```python
from build123d import *

# Parameters (mm, degrees)
BOSS_EXTRU_1_DEPTH                                 = 5
ESQUISSE7_W                                        = 36
ESQUISSE7_H                                        = 2
BOSS_EXTRU_2_DEPTH                                 = 35
BOSS_EXTRU_4_DEPTH                                 = 4
ESQUISSE1_3_R                                      = 6.5
ENL_V_MAT_EXTRU_2_DEPTH                            = 63.737548565
CHAMBRAGE_POUR_VIS_T_TE_HEXAGONALE_M41_D           = 4.5
CHAMBRAGE_POUR_VIS_T_TE_HEXAGONALE_M41_DEPTH       = 4
CHAMBRAGE_POUR_VIS_T_TE_HEXAGONALE_M41_CBORE_D     = 10.59
CHAMBRAGE_POUR_VIS_T_TE_HEXAGONALE_M41_CBORE_DEPTH = 3
CHAMBRAGE_POUR_VIS_T_TE_HEXAGONALE_M41_TIP         = 1.351936393
CONG_1_R                                           = 5
CONG_2_R                                           = 7


with BuildPart() as part:
    # Esquisse1 → Boss.-Extru.1 (new body)
    with BuildSketch(Plane(origin=(0, 0, 0), x_dir=(1, 0, 0), z_dir=(0, 1, 0))):
        with BuildLine():
            Line((20, 20), (-20, 20))
            Line((-20, 20), (-20, -3.067363788))
            ThreePointArc((-20, -3.067363788), (-23.03, -8), (-20, -12.932636212))
            Line((-20, -12.932636212), (-20, -20))
            Line((-20, -20), (20, -20))
            Line((20, -20), (20, -12.932636212))
            ThreePointArc((20, -12.932636212), (23.03, -8), (20, -3.067363788))
            Line((20, -3.067363788), (20, 20))
        make_face()
        with BuildLine():
            ThreePointArc((-16.580993336, -9.888233765), (-17.5, -10.1), (-18.419006664, -9.888233765))
            ThreePointArc((-18.419006664, -9.888233765), (-18.799038106, -8.75), (-19.594761741, -7.851766235))
            ThreePointArc((-19.594761741, -7.851766235), (-19.318653348, -6.95), (-18.675755077, -6.26))
            ThreePointArc((-18.675755077, -6.26), (-17.5, -6.5), (-16.324244923, -6.26))
            ThreePointArc((-16.324244923, -6.26), (-15.681346652, -6.95), (-15.405238259, -7.851766235))
            ThreePointArc((-15.405238259, -7.851766235), (-16.200961894, -8.75), (-16.580993336, -9.888233765))
        make_face(mode=Mode.SUBTRACT)
        with BuildLine():
            Line((4.596194078, -4.596194078), (0, -9.192388155))
            Line((0, -9.192388155), (-4.596194078, -4.596194078))
            ThreePointArc((-4.596194078, -4.596194078), (0, 6.5), (4.596194078, -4.596194078))
        make_face(mode=Mode.SUBTRACT)
        with BuildLine():
            ThreePointArc((18.419006664, -9.888233765), (17.5, -10.1), (16.580993336, -9.888233765))
            ThreePointArc((16.580993336, -9.888233765), (16.200961894, -8.75), (15.405238259, -7.851766235))
            ThreePointArc((15.405238259, -7.851766235), (15.681346652, -6.95), (16.324244923, -6.26))
            ThreePointArc((16.324244923, -6.26), (17.5, -6.5), (18.675755077, -6.26))
            ThreePointArc((18.675755077, -6.26), (19.318653348, -6.95), (19.594761741, -7.851766235))
            ThreePointArc((19.594761741, -7.851766235), (18.799038106, -8.75), (18.419006664, -9.888233765))
        make_face(mode=Mode.SUBTRACT)
    extrude(amount=-BOSS_EXTRU_1_DEPTH)

    # Esquisse7 → Boss.-Extru.2 (add)
    with BuildSketch(Plane.XZ.offset(5)):
        Polygon((-20, 2.243441463), (-20, -20), (-18, -20), (-18, -18), (-18, 2.243441463), align=None)
        with Locations((0, -19)):
            Rectangle(ESQUISSE7_W, ESQUISSE7_H)
        Polygon((18, -18), (18, -20), (20, -20), (20, 2.243441463), (18, 2.243441463), align=None)
    extrude(amount=BOSS_EXTRU_2_DEPTH)

    # Esquisse9 → Boss.-Extru.4 (add)
    with BuildSketch(Plane.XZ.offset(40)):
        Polygon((-20, 2.243441463), (-20, 20), (-40, 20), (-40, -20), (-20, -20), align=None)
        Polygon((40, 20), (20, 20), (20, 2.243441463), (20, -20), (40, -20), align=None)
        Polygon((0, -18), (0, 20), (-20, 20), (-20, 2.243441463), (-18, 2.243441463), (-18, -18), align=None)
        Polygon((0, -20), (0, -18), (-18, -18), (-18, 2.243441463), (-20, 2.243441463), (-20, -20), align=None)
        Polygon((18, -18), (0, -18), (0, -20), (20, -20), (20, 2.243441463), (18, 2.243441463), align=None)
        Polygon((20, 20), (0, 20), (0, -18), (18, -18), (18, 2.243441463), (20, 2.243441463), align=None)
    extrude(amount=BOSS_EXTRU_4_DEPTH)

    # Esquisse1<3> → Enlèv. mat.-Extru.2 (cut, through all)
    with BuildSketch(Plane(origin=(0, 0, 0), x_dir=(1, 0, 0), z_dir=(0, 1, 0))):
        Circle(ESQUISSE1_3_R)
        with BuildLine():
            Line((0, -9.192388155), (4.596194078, -4.596194078))
            ThreePointArc((4.596194078, -4.596194078), (0, -6.5), (-4.596194078, -4.596194078))
            Line((-4.596194078, -4.596194078), (0, -9.192388155))
        make_face()
    extrude(amount=-ENL_V_MAT_EXTRU_2_DEPTH, mode=Mode.SUBTRACT)

    # Chambrage pour vis à tête hexagonale M41
    with Locations(Plane(origin=(0, -40, 0), x_dir=(1, 0, 0), z_dir=(0, 1, 0))):
        with Locations((-32, -12), (-32, 12), (32, 12), (32, -12)):
            CounterBoreHole(CHAMBRAGE_POUR_VIS_T_TE_HEXAGONALE_M41_D / 2, CHAMBRAGE_POUR_VIS_T_TE_HEXAGONALE_M41_CBORE_D / 2, CHAMBRAGE_POUR_VIS_T_TE_HEXAGONALE_M41_CBORE_DEPTH, depth=CHAMBRAGE_POUR_VIS_T_TE_HEXAGONALE_M41_DEPTH)
            with Locations((0, 0, -(CHAMBRAGE_POUR_VIS_T_TE_HEXAGONALE_M41_DEPTH + CHAMBRAGE_POUR_VIS_T_TE_HEXAGONALE_M41_TIP / 2))):  # 118° drill point
                Cone(0, CHAMBRAGE_POUR_VIS_T_TE_HEXAGONALE_M41_D / 2, CHAMBRAGE_POUR_VIS_T_TE_HEXAGONALE_M41_TIP, mode=Mode.SUBTRACT)

    # Congé1
    cong_1_edges = [part.edges().sort_by_distance(p)[0] for p in [
        (18, -22.5, -18),
        (-18, -22.5, -18),
    ]]
    fillet(cong_1_edges, radius=CONG_1_R)

    # Congé2
    cong_2_edges = [part.edges().sort_by_distance(p)[0] for p in [
        (-20, -20, -20),
        (20, -20, -20),
        (20, -2.5, 20),
        (-20, -2.5, 20),
    ]]
    fillet(cong_2_edges, radius=CONG_2_R)


solid = part.part
```
Work out the finished part from the listing and answer in its coordinate system (mm). A direction names the side the tool comes from. Give positions to 0.01 mm unless a question says otherwise; leave off trailing zeros. Write each loop counter-clockwise with the first axis right and the second up, starting at its lowest first coordinate (ties: lowest second). Pieces come first, ordered by that corner, then holes.
(1) Flat-ended cylindrical pins translate along their axes: pin 1 Ø8 at (x, y) = (12.5, -18.5) entering from +Z; pin 2 Ø8 at (y, z) = (-25.5, -3.5) entering from +X; pin 3 Ø4 at (x, z) = (-32, -12) entering from +Y; pin 4 Ø8 at (x, y) = (-2, -27.5) entering from +Z. Find the tip coordinate at first contact, or state that the pin passes through.
Final values:
pin 1: stops at z = -16.57
pin 2: stops at x = 20
pin 3: passes through
pin 4: stops at z = -18
(2) The part is cut by section D-D on y = -22. Write down the section's boundary in (x, z).
Final values:
outline: (-20, -13) arc R7 ccw to (-13, -20) - (13, -20) arc R7 ccw to (20, -13) - (20, 2.24) - (18, 2.24) - (18, -13) arc R5 cw to (13, -18) - (-13, -18) arc R5 cw to (-18, -13) - (-18, 2.24) - (-20, 2.24) - close
(3) The part is cut by section B-B on x = -32. Write down the section's boundary in (y, z) (3 decimals).
Final values:
outline: (-44, -20) - (-40, -20) - (-40, -17.295) - (-43, -17.295) - (-43, -14.25) - (-44, -14.25) - close; (-44, -9.75) - (-43, -9.75) - (-43, -6.705) - (-40, -6.705) - (-40, 6.705) - (-43, 6.705) - (-43, 9.75) - (-44, 9.75) - close; (-44, 14.25) - (-43, 14.25) - (-43, 17.295) - (-40, 17.295) - (-40, 20) - (-44, 20) - close
(4) The mould has two halves that part along X. Classify faces 1 (the flat face through (-1, -27, -20)), 2 (the cylindrical face through (17.9, -2.5, 18)), 3 (the flat face through (2.33, -2.46, 6.86)): pulls with the +X half, pulls with the -X half, needs draft (parallel to the pull), parting line crosses it, or undercut.
Final values:
face 1: needs draft
face 2: pulls with the +X half
face 3: undercut
(5) Which of the six approach directions +Z, -Z, +X, -X, +Y, -Y give full straight-line access (tool end or side, diameter ignored) to faces 4 (the cylindrical face through (-0.214, -2.465, -6.496)), 5 (the cylindrical face through (16, -23, -17)), 6 (the cylindrical face through (17.5, -2.5, 6.5))?
Final values:
face 4: +Y, -Y
face 5: +Z
face 6: +Y
(6) Straight lines are drawn through the part: line 1 (X direction, y = -12, z = 1.5); line 2 (Z direction, x = -32, y = -43.65); line 3 (Y direction, x = -14, z = 17). For each, find the intervals that lie inside material, in ascending order.
Final values:
line 1: x = -20 to -18, 18 to 20
line 2: z = -20 to -14.25, -9.75 to 9.75, 14.25 to 20
line 3: y = -44 to -40, -5 to 0
(7) The part is cut by section A-A on z = -12. Write down the section's boundary in (x, y) (3 decimals).
Final values:
outline: (-40, -44) - (-34.25, -44) - (-34.25, -43) - (-37.295, -43) - (-37.295, -40) - (-40, -40) - close; (-29.75, -44) - (29.75, -44) - (29.75, -43) - (26.705, -43) - (26.705, -40) - (20, -40) - (20, 0) - (-20, 0) - (-20, -40) - (-26.705, -40) - (-26.705, -43) - (-29.75, -43) - close; (34.25, -44) - (40, -44) - (40, -40) - (37.295, -40) - (37.295, -43) - (34.25, -43) - close; hole (-18, -40) - (18, -40) - (18, -5) - (-18, -5) - close
(8) The part is cut by section C-C on x = 12. Write down the section's boundary in (y, z).
Final values:
outline: (-44, -20) - (0, -20) - (0, 20) - (-5, 20) - (-5, -18) - (-40, -18) - (-40, 20) - (-44, 20) - close
